Source: CAD feature listing. Evaluate the final solid. Frame: model axes, mm. Give positions to 0.01 mm unless a question says otherwise; leave off trailing zeros. Loops run counter-clockwise (first coordinate to the right, second up) from the corner with the lowest first, then second, coordinate; pieces in that order, holes last.
from build123d import *

# Parameters (mm, degrees)
SKIZZE1_W                            = 326
SKIZZE1_H                            = 50
AUFSATZ_LINEAR_AUSTRAGEN1_DEPTH      = 3
DURCHGANGSLOCH_F_R_M41_D             = 4.5
F_9_0_12_DURCHMESSER_BOHRUNG1_D      = 12
FORMSENKUNG_F_R_M4_SFHCS1_AT_2_COUNT = 2
FORMSENKUNG_F_R_M4_SFHCS1_AT_2_PITCH = 306
FORMSENKUNG_F_R_M4_SFHCS1_AT_3_COUNT = 2
FORMSENKUNG_F_R_M4_SFHCS1_AT_3_PITCH = 282.596886041
FORMSENKUNG_F_R_M4_SFHCS1_AT_4_COUNT = 2
FORMSENKUNG_F_R_M4_SFHCS1_AT_4_PITCH = 185.442713526
FORMSENKUNG_F_R_M4_SFHCS1_AT_5_COUNT = 2
FORMSENKUNG_F_R_M4_SFHCS1_AT_5_PITCH = 126.605687076
FORMSENKUNG_F_R_M4_SFHCS1_AT_6_COUNT = 2
FORMSENKUNG_F_R_M4_SFHCS1_AT_6_PITCH = 39.05124838


with BuildPart() as part:
    # Skizze1 → Aufsatz-Linear austragen1 (new body)
    with BuildSketch(Plane(origin=(0, 0, 0), x_dir=(1, 0, 0), z_dir=(0, 1, 0))):
        Rectangle(SKIZZE1_W, SKIZZE1_H)
    extrude(amount=AUFSATZ_LINEAR_AUSTRAGEN1_DEPTH)

    # Durchgangsloch für M41 (through all)
    with Locations(Plane(origin=(0, 3, 0), x_dir=(1, 0, 0), z_dir=(0, 1, 0))):
        with Locations((0, 0), (0, 10)):
            Hole(DURCHGANGSLOCH_F_R_M41_D / 2)

    # Ø9.0 (12) Durchmesser Bohrung1 (through all)
    with Locations(Plane(origin=(0, 3, 0), x_dir=(1, 0, 0), z_dir=(0, 1, 0))):
        with Locations((-95.5, 5), (95.5, 5)):
            Hole(F_9_0_12_DURCHMESSER_BOHRUNG1_D / 2)

    # Skizze7 → Formsenkung für M4 SFHCS1 (revolve, cut)
    with BuildSketch(Plane(origin=(153, 0, -15), x_dir=(0, 0, -1), z_dir=(1, 0, 0))):
        Polygon((0, 0), (0, 3), (2.25, 3), (2.25, 2.23), (4.48, 0), align=None)
    formsenkung_f_r_m4_sfhcs1 = revolve(axis=Axis((153, -6.35, -15), (0, 1, 0)), mode=Mode.SUBTRACT)

    # Formsenkung für M4 SFHCS1 at 2: Formsenkung für M4 SFHCS1 ×2
    with Locations(*[(-i * FORMSENKUNG_F_R_M4_SFHCS1_AT_2_PITCH, 0, 0) for i in range(1, FORMSENKUNG_F_R_M4_SFHCS1_AT_2_COUNT)]):
        add(formsenkung_f_r_m4_sfhcs1, mode=Mode.SUBTRACT)

    # Formsenkung für M4 SFHCS1 at 3: Formsenkung für M4 SFHCS1 ×2
    with Locations(*[Vector(-0.9943492440300802, 0, 0.10615828228079148) * (i * FORMSENKUNG_F_R_M4_SFHCS1_AT_3_PITCH) for i in range(1, FORMSENKUNG_F_R_M4_SFHCS1_AT_3_COUNT)]):
        add(formsenkung_f_r_m4_sfhcs1, mode=Mode.SUBTRACT)

    # Formsenkung für M4 SFHCS1 at 4: Formsenkung für M4 SFHCS1 ×2
    with Locations(*[Vector(-0.9868276651055338, 0, 0.16177502706648092) * (i * FORMSENKUNG_F_R_M4_SFHCS1_AT_4_PITCH) for i in range(1, FORMSENKUNG_F_R_M4_SFHCS1_AT_4_COUNT)]):
        add(formsenkung_f_r_m4_sfhcs1, mode=Mode.SUBTRACT)

    # Formsenkung für M4 SFHCS1 at 5: Formsenkung für M4 SFHCS1 ×2
    with Locations(*[Vector(-0.9715203387831296, 0, 0.23695618019100717) * (i * FORMSENKUNG_F_R_M4_SFHCS1_AT_5_PITCH) for i in range(1, FORMSENKUNG_F_R_M4_SFHCS1_AT_5_COUNT)]):
        add(formsenkung_f_r_m4_sfhcs1, mode=Mode.SUBTRACT)

    # Formsenkung für M4 SFHCS1 at 6: Formsenkung für M4 SFHCS1 ×2
    with Locations(*[Vector(-0.6401843996644799, 0, 0.7682212795973759) * (i * FORMSENKUNG_F_R_M4_SFHCS1_AT_6_PITCH) for i in range(1, FORMSENKUNG_F_R_M4_SFHCS1_AT_6_COUNT)]):
        add(formsenkung_f_r_m4_sfhcs1, mode=Mode.SUBTRACT)


solid = part.part
1) Contact query for flat-ended pins moving along their axis: P1, Ø6, axis at x = 153, z = -15, coming from the -Y side; P2, Ø7, axis at x = -128, z = 15, coming from the -Y side. Output: stop coordinate, or through.
Checks:
P1: stops at y = 1.48
P2: stops at y = 0.98
2) Pull-direction query (Z, two-part tool) for faces 1 (the flat face through (-2, 3, -6)), 2 (the conical face through (-150.67, 2.09, -14.48)); classes: released by +Z, released by -Z, zero draft, split by the parting line, or undercut.
Checks:
face 1: zero draft
face 2: undercut
3) Cut plane B-B (z = -5). Return loops of the section in (x, y), and give its area (3 significant figures).
Checks:
outline: (-163, 0) - (-101.5, 0) - (-101.5, 3) - (-163, 3) - close; (-89.5, 0) - (89.5, 0) - (89.5, 3) - (-89.5, 3) - close; (101.5, 0) - (163, 0) - (163, 3) - (101.5, 3) - close
area: 906 mm2
4) Ray query, probe 1 along X at (y, z) = (2.75, 15); probe 2 along X at (y, z) = (2.5, -15); probe 3 along Z at (x, y) = (-128, 2.7). Return the intervals inside material, ascending.
Checks:
probe 1: x = -163 to -130.25, -125.75 to -32.25, -27.75 to 27.75, 32.25 to 125.75, 130.25 to 163
probe 2: x = -163 to -155.25, -150.75 to 150.75, 155.25 to 163
probe 3: z = -25 to 12.75, 17.25 to 25
5) Cut plane A-A (y = 1.3). State how many separate pieces and enclosed holes the cut face has, and give its area (3 significant figures).
Checks:
separate pieces: 1
enclosed holes: 10
area: 15,900 mm2
